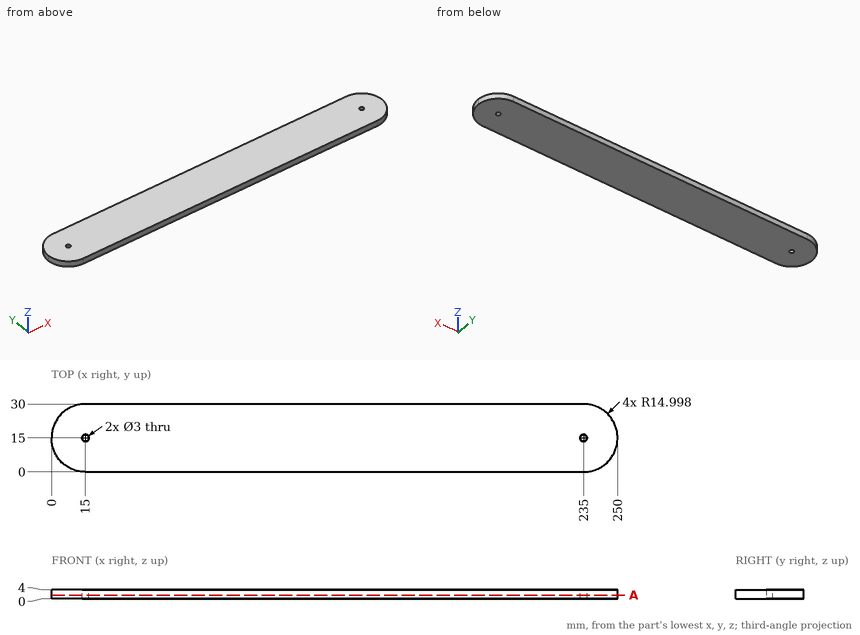
Geometry: see drawing. Coordinates: mm, zero at the bounding-box minimum. Round coordinates to 2 decimals unless told otherwise and drop trailing zeros.
1) Cut plane A-A (z = 1.7). Count the separate pieces of the cut face and the enclosed holes in it, then the cut area to 3 significant figures.
2) Contact query for flat-ended pins moving along their axis: P1, Ø1, axis at y = 14, z = 1.5, coming from the +X side; P2, Ø2, axis at y = 23.5, z = 0.5, coming from the -X side; P3, Ø2.5, axis at x = 15, y = 15, coming from the -Z side. Output: stop coordinate, or through.
3) Ray query, L1, parallel to X at y = 15, z = 2.3; L2, parallel to Y at x = 15, z = 2.7; L3, parallel to Y at x = 15.5, z = 0.6 (1 decimal). Return the intervals inside material, ascending.
Geometry says:
1. separate pieces: 1
1. enclosed holes: 2
1. area: 7,290 mm2
2. P1: stops at x = 249.99
2. P2: stops at x = 2.01
2. P3: passes through
3. L1: x = 0 to 13.5, 16.5 to 233.5, 236.5 to 250
3. L2: y = 0 to 13.5, 16.5 to 30
3. L3: y = 0 to 13.6, 16.4 to 30
